Here's how the part is built. I have some questions about the finished solid (model axes, mm). A direction names the side the tool comes from. Round coordinates to 2 decimals unless told otherwise and drop trailing zeros. Loops run counter-clockwise (first coordinate to the right, second up) from the corner with the lowest first, then second, coordinate; pieces in that order, holes last. Notation, with made-up numbers: M 81,15.25 L 114,15.25 A21 cw 114,45.25 Z; hole C 35.25,-25 d2. An arc over 180 degrees is marked long. Answer as a JSON object with one key per item and string values.
from build123d import *

# Parameters (mm, degrees)
BOSS_EXTRUDE1_DEPTH = 83.125
SKETCH2_W           = 25.914253455
SKETCH2_H           = 3.3
BOSS_EXTRUDE2_DEPTH = 10


with BuildPart() as part:
    # Sketch1 → Boss-Extrude1 (new body)
    with BuildSketch(Plane(origin=(0, 0, 0), x_dir=(-1, 0, 0), z_dir=(0, 1, 0))):
        Polygon((69.688093764, 147.570616058), (29.688093764, 147.570616058), (39.245883851, 144.62975757), (37.073840309, 137.570616058), (69.688093764, 137.570616058), align=None)
        Polygon((39.245883851, 144.62975757), (29.688093764, 147.570616058), (29.688093764, 137.570616058), (37.073840309, 137.570616058), align=None)
        Polygon((29.688093764, 147.570616058), (-10.311906236, 17.570616058), (-5.311906236, 17.570616058), (0.150763386, 17.570616058), (37.073840309, 137.570616058), (29.688093764, 137.570616058), align=None)
        Polygon((-5.311906236, 16.03215452), (-10.311906236, 17.570616058), (-10.311906236, 10.070616058), (-5.311906236, 10.070616058), align=None)
        Polygon((-5.311906236, 17.570616058), (-10.311906236, 17.570616058), (-5.311906236, 16.03215452), align=None)
    extrude(amount=BOSS_EXTRUDE1_DEPTH)

    # Sketch2 → Boss-Extrude2 (add)
    with BuildSketch(Plane(origin=(0, 83.125, 0), x_dir=(-1, 0, 0), z_dir=(0, 1, 0))):
        Polygon((32.886793036, 135.353943973), (-2.0659087, 21.757663331), (-5.219979428, 22.728146632), (29.732722307, 136.324427274), align=None)
        with Locations((53.380967037, 142.570616058)):
            Rectangle(SKETCH2_W, SKETCH2_H)
    boss_extrude2 = extrude(amount=BOSS_EXTRUDE2_DEPTH)

    # Mirror1: Boss-Extrude2 across plane
    add(boss_extrude2.mirror(Plane.ZX.offset(41.5625)))


solid = part.part
Item 1: I want a section at B-B, the plane x = -51. Please give me the cut outline in (y, z) (3 decimals), then the cut area to 3 significant figures.
Resolved:
{"outline": "M -10,140.921 L 0,140.921 L 0,137.571 L 83.125,137.571 L 83.125,140.921 L 93.125,140.921 L 93.125,144.221 L 83.125,144.221 L 83.125,147.571 L 0,147.571 L 0,144.221 L -10,144.221 Z", "area": "897 mm²"}
Item 2: On a 3-axis mill with a long thin cutter (end or side, diameter ignored), from which of +Z, -Z, +X, -X, +Y, -Y can I reach the whole of each face in a straight line? I mean faces 1 (the face through (-66.338, 88, 143)), 2 (the face through (-31.288, -4.93, 135.846)), 3 (the face through (5.312, 41, 14)), 4 (the face through (-66.338, -5, 143)), 5 (the face through (-40.424, 88, 143)). Say none if no direction works.
Resolved:
{"face 1": "+Z, -Z, -X, +Y", "face 2": "+Z, -X, -Y", "face 3": "-Z, -X, +Y, -Y", "face 4": "+Z, -Z, -X, -Y", "face 5": "+Z, -Z, +X, +Y"}
Item 3: I want a section at A-A, the plane y = -2. Please give me the cut outline in (x, z).
Resolved:
{"outline": "M -66.34,140.92 L -40.42,140.92 L -40.42,144.22 L -66.34,144.22 Z; M -32.89,135.35 L 2.07,21.76 L 5.22,22.73 L -29.73,136.32 Z"}
Item 4: Please list where these lines run through material, in increasing order: probe 1 along Z at (x, y) = (-57, 13); probe 2 along Y at (x, z) = (-14, 66) (3 decimals); probe 3 along X at (y, z) = (70.5, 88). Write a range as from..to.
Resolved:
{"probe 1": "137.57..147.57", "probe 2": "0..83.125", "probe 3": "-21.82..-11.36"}
Item 5: I want a section at D-D, the plane z = 29. Please give me the cut outline in (x, y) (1 decimal).
Resolved:
{"outline": "M -3.7,0 L -0.2,0 L -0.2,-10 L 3.3,-10 L 3.3,0 L 6.8,0 L 6.8,83.1 L 3.3,83.1 L 3.3,93.1 L -0.2,93.1 L -0.2,83.1 L -3.7,83.1 Z"}
Item 6: I'm going to push flat-ended pins straight in: pin 1 Ø1 at (y, z) = (88.5, 143) entering from -X; pin 2 Ø2.5 at (x, y) = (2.5, 28) entering from -Z; pin 3 Ø3.5 at (y, z) = (-6.5, 142) entering from +X. Where does each tip first touch, or does it pass through?
Resolved:
{"pin 1": "x = -66.34", "pin 2": "z = 17.57", "pin 3": "x = -40.42"}
Item 7: I want a section at C-C, the plane y = 55.5. Please give me the cut outline in (x, z), then the cut area to 3 significant figures.
Resolved:
{"outline": "M -69.69,137.57 L -37.07,137.57 L -0.15,17.57 L 5.31,17.57 L 5.31,10.07 L 10.31,10.07 L 10.31,17.57 L -29.69,147.57 L -69.69,147.57 Z", "area": "1,710 mm²"}
